Geometry check sheet. Reference: the model listing, model coordinates, mm. A direction names the side the tool comes from. Coordinates: 2 decimals unless noted, no trailing zeros. Order: outer loops, then holes, each group sorted by start corner. A loop starts at its lowest first (then second) coordinate and runs counter-clockwise, first axis right, second up. Notation, with made-up numbers: (-7.5, -37.75) - (7.5, -37.75) arc R12 ccw to (7.5, -26.75) - close; hole circle Ø8 at (-29, -28). An arc over 180 degrees is marked (long way). One line per item, written item: value. Start each with the question number.
```python
from build123d import *

# Parameters (mm, degrees)
F0_W      = 50.8
F0_H      = 50.8
F1_DEPTH  = 50.8
F2_R      = 9
F3_DEPTH  = 407.416
F4_W      = 60.1204171121
F4_H      = 25.4
F5_DEPTH  = 338.582
F6_R      = 5.08
F7_DEPTH  = 5.08
F8_R      = 2.159
F9_DEPTH  = 25.4
F10_R     = 1.5494
F11_DEPTH = 25.4
F12_R     = 1.5494
F12_R_2   = 2.159
F13_DEPTH = 25.4
F18_DEPTH = 72.39
F21_R     = 12.7


with BuildPart() as f1:
    # F0 (on Top) → F1 (new body)
    with BuildSketch(Plane.XY):
        Rectangle(F0_W, F0_H)
    extrude(amount=F1_DEPTH)

    # F2 (on face) → F3 (cut)
    with BuildSketch(Plane(origin=(0, 0, 0), x_dir=(1, 0, 0), z_dir=(0, 0, -1))):
        Circle(F2_R)
    extrude(amount=-F3_DEPTH, mode=Mode.SUBTRACT)

    # F4 (on face) → F5 (cut)
    with BuildSketch(Plane(origin=(0, 0, 0), x_dir=(1, 0, 0), z_dir=(0, 0, -1))):
        with Locations((4.6602085561, 12.7)):
            Rectangle(F4_W, F4_H)
    extrude(amount=-F5_DEPTH, mode=Mode.SUBTRACT)

    # F6 (on face) → F7 (cut)
    with BuildSketch(Plane.XZ):
        with Locations((-17.2, 25.4)):
            Circle(F6_R)
    extrude(amount=-F7_DEPTH, mode=Mode.SUBTRACT)

    # F8 (on face) → F9 (cut)
    with BuildSketch(Plane.XZ.offset(-5.08)):
        with Locations((-17.2, 25.4)):
            Circle(F8_R)
    extrude(amount=-F9_DEPTH, mode=Mode.SUBTRACT)

    # F10 (on face) → F11 (cut)
    with BuildSketch(Plane.XZ):
        with Locations((-17.2, 44.4713309407)):
            Circle(F10_R)
    extrude(amount=-F11_DEPTH, mode=Mode.SUBTRACT)

    # F12 (on face) → F13 (cut)
    with BuildSketch(Plane.XZ):
        with Locations((17.2, 44.4713309407)):
            Circle(F12_R)
        with Locations((17.2, 25.4)):
            Circle(F12_R_2)
    extrude(amount=-F13_DEPTH, mode=Mode.SUBTRACT)

    # F16: F1 across plane


with BuildPart() as f1_1:
    add(f1.part)
    add(f1.part.mirror(Plane(origin=(0, 13.6714489466, 25.4), x_dir=(1, 0, 0), z_dir=(0, 0, 1))), mode=Mode.INTERSECT)

    # F17 (on face) → F18 (cut)
    with BuildSketch(Plane(origin=(0, 0, 0), x_dir=(1, 0, 0), z_dir=(0, 0, -1))):
        Polygon((37.3146161437, -15.35), (0, -15.35), (-44.7141490877, -15.35), (-42.6479764283, -31.9298505783), (43.3826521039, -33.9571945369), align=None)
    extrude(amount=-F18_DEPTH, mode=Mode.SUBTRACT)

    # F21
    f21_edges = [f1_1.edges().sort_by_distance(p)[0] for p in [
        (25.4, 7.675, 50.8),
        (25.4, 7.675, 0),
        (-25.4, 7.675, 50.8),
        (-25.4, 7.675, 0),
    ]]
    fillet(f21_edges, radius=F21_R)


solid = f1_1.part
```
Q1. Cross-section at C-C, the plane y = 11. Enter the section's corners in (x, z), and give its area (3 significant figures).
Q2. Material ranges on probe 1 along Z at (x, y) = (18.5, 4.5); probe 2 along Z at (x, y) = (-17.2, 1.9); probe 3 along X at (y, z) = (3.25, 5.5), recorded low to high.
Q3. Cross-section at D-D, the plane x = 0. Enter the section's corners in (y, z), and give its area (3 significant figures).
Q4. Set-up check for faces 4 (the flat face through (-0.2, 9.5, 50.8)), 5 (the flat face through (-17, 5.08, 23)): record each of +Z, -Z, +X, -X, +Y, -Y from which the full face is reachable in a straight line by a thin tool's end or side.
Q5. Cross-section at B-B, the plane z = 24. Enter the section's corners in (x, y), and give its area (3 significant figures).
Q6. Release check for a two-part mould opening along Z. For faces 1 (the cylindrical face through (21.58, 7.78, 3.62)), 2 (the cylindrical face through (-20.944, 2.504, 28.833)), 3 (the flat face through (13, 0, 25)) record: released by +Z, released by -Z, zero draft, split by the parting line, or undercut.
Q7. Cross-section at A-A, the plane y = 2.25. Enter the section's corners in (x, z).
Q8. Gauge pin test, flat end, axial feed: P1, Ø7, axis at x = 17.2, z = 25.4, coming from the +Y side. Record the tip position at first contact, or that the pin passes through.
Check result:
1. outline: (-25.4, 12.7) arc R12.7 ccw to (-12.7, 0) - (12.7, 0) arc R12.7 ccw to (25.4, 12.7) - (25.4, 38.1) arc R12.7 ccw to (12.7, 50.8) - (-12.7, 50.8) arc R12.7 ccw to (-25.4, 38.1) - close; hole circle Ø4.32 at (-17.2, 25.4); hole circle Ø3.1 at (-17.2, 6.33); hole circle Ø3.1 at (-17.2, 44.47); hole circle Ø4.32 at (17.2, 25.4); hole circle Ø3.1 at (17.2, 6.33); hole circle Ø3.1 at (17.2, 44.47)
1. area: 2,380 mm2
2. probe 1: z = 1.4 to 5.49, 7.17 to 23.68, 27.12 to 43.63, 45.31 to 49.4
2. probe 2: z = 0.82 to 4.78, 7.88 to 20.32, 30.48 to 42.92, 46.02 to 49.98
2. probe 3: x = -23.16 to -18.51, -15.89 to -8.39, 8.39 to 15.89, 18.51 to 23.16
3. outline: (9, 0) - (15.35, 0) - (15.35, 50.8) - (9, 50.8) - close
3. area: 323 mm2
4. face 4: +Z, +X, -X, +Y, -Y
4. face 5: -Y
5. outline: (-25.4, 0) - (-22.08, 0) - (-22.08, 5.08) - (-18.84, 5.08) - (-18.84, 15.35) - (-25.4, 15.35) - close; (-15.56, 5.08) - (-12.32, 5.08) - (-12.32, 0) - (-9, 0) arc R9 cw to (9, 0) - (15.56, 0) - (15.56, 15.35) - (-15.56, 15.35) - close; (18.84, 0) - (25.4, 0) - (25.4, 15.35) - (18.84, 15.35) - close
5. area: 519 mm2
6. face 1: released by -Z
6. face 2: undercut
6. face 3: zero draft
7. outline: (-25.4, 12.7) arc R12.7 ccw to (-12.7, 0) - (-8.71, 0) - (-8.71, 50.8) - (-12.7, 50.8) arc R12.7 ccw to (-25.4, 38.1) - close; (8.71, 0) - (12.7, 0) arc R12.7 ccw to (25.4, 12.7) - (25.4, 38.1) arc R12.7 ccw to (12.7, 50.8) - (8.71, 50.8) - close; hole circle Ø10.16 at (-17.2, 25.4); hole circle Ø3.1 at (-17.2, 6.33); hole circle Ø3.1 at (-17.2, 44.47); hole circle Ø4.32 at (17.2, 25.4); hole circle Ø3.1 at (17.2, 6.33); hole circle Ø3.1 at (17.2, 44.47)
8. P1: stops at y = 15.35
